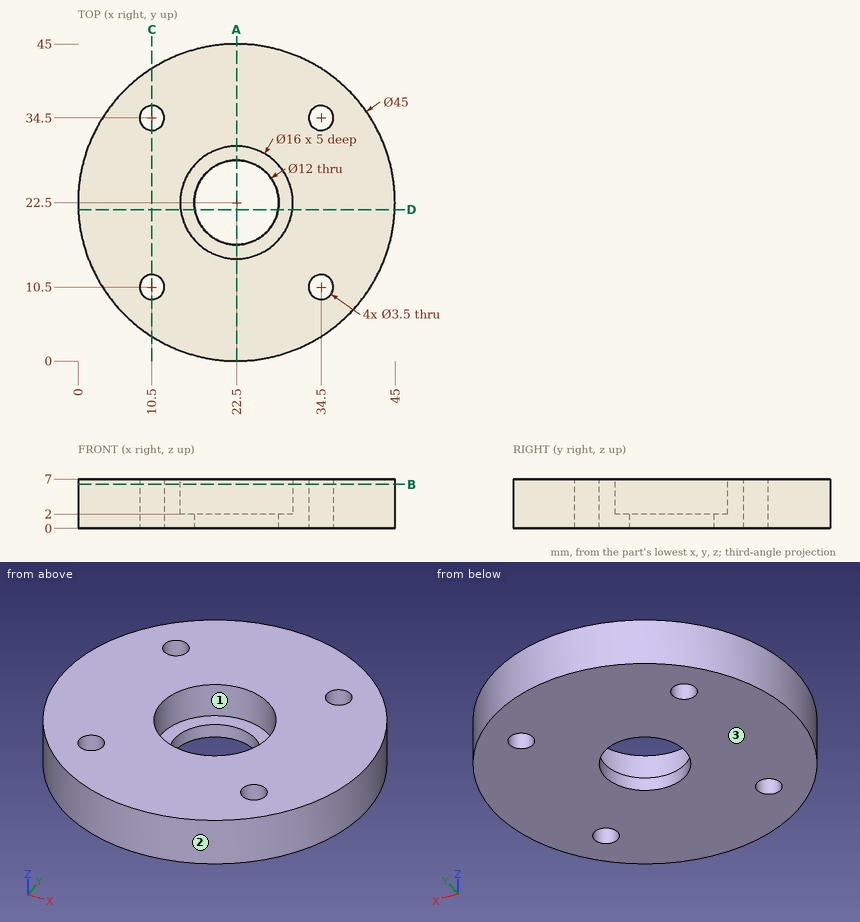
Print and shaded views of the part. All mm, measured from the part's lowest x, y and z. Coordinates: 2 decimals unless noted, no trailing zeros. Loops run counter-clockwise (first coordinate to the right, second up) from the corner with the lowest first, then second, coordinate; pieces in that order, holes last. Notation, with made-up numbers: (78.25, -9.75) - (131.25, -9.75) arc R25 cw to (131.25, 24.25) - close; hole circle Ø3 at (-37, 9). An arc over 180 degrees is marked (long way). Write item = value, one per line. Start each with the question number.
Item 1: Wall check: probe 1 along Y at (x, z) = (10.5, 2.25); probe 2 along Y at (x, z) = (9.5, 2.75); probe 3 along X at (y, z) = (33, 5). Give the ranges that are in metal, low to high. Write a range as [from, to].
Item 2: Saw through at C-C, the plane x = 10.5. List the corners of the cut face in (y, z).
Item 3: Saw through at A-A, the plane x = 22.5. List the corners of the cut face in (y, z), then the cut area to 3 significant figures.
Item 4: Saw through at D-D, the plane y = 21.5. List the corners of the cut face in (x, z), then the cut area to 3 significant figures.
Item 5: Saw through at B-B, the plane z = 6.25. List the corners of the cut face in (x, y), then the cut area to 3 significant figures.
Item 6: Pull direction X, two halves, no side cores. Call the marked faces 1, 2 and 3: +X half, -X half, draft (parallel to the pull), parting line (faces both ways), or undercut.
Item 7: Drop flat-ended pins along their axis: pin 1 Ø2 at (x, y) = (34.5, 34.5) entering from -Z; pin 2 Ø4 at (x, z) = (16, 6) entering from -Y; pin 3 Ø2 at (y, z) = (35, 2) entering from +X. Give the stop position or say it passes through.
Answers:
q1.probe_1 = [3.47, 8.75], [12.25, 32.75], [36.25, 41.53]
q1.probe_2 = [4.14, 9.06], [11.94, 33.06], [35.94, 40.86]
q1.probe_3 = [2.6, 9.6], [11.4, 33.6], [35.4, 42.4]
q2.outline = (3.47, 0) - (8.75, 0) - (8.75, 7) - (3.47, 7) - close; (12.25, 0) - (32.75, 0) - (32.75, 7) - (12.25, 7) - close; (36.25, 0) - (41.53, 0) - (41.53, 7) - (36.25, 7) - close
q3.outline = (0, 0) - (16.5, 0) - (16.5, 2) - (14.5, 2) - (14.5, 7) - (0, 7) - close; (28.5, 0) - (45, 0) - (45, 7) - (30.5, 7) - (30.5, 2) - (28.5, 2) - close
q3.area = 211 mm2
q4.outline = (0.02, 0) - (16.58, 0) - (16.58, 2) - (14.56, 2) - (14.56, 7) - (0.02, 7) - close; (28.42, 0) - (44.98, 0) - (44.98, 7) - (30.44, 7) - (30.44, 2) - (28.42, 2) - close
q4.area = 212 mm2
q5.outline = circle Ø45 at (22.5, 22.5); hole circle Ø3.5 at (10.5, 10.5); hole circle Ø3.5 at (10.5, 34.5); hole circle Ø16 at (22.5, 22.5); hole circle Ø3.5 at (34.5, 10.5); hole circle Ø3.5 at (34.5, 34.5)
q5.area = 1,350 mm2
q6.face_1 = undercut
q6.face_2 = parting line
q6.face_3 = draft
q7.pin_1 = through
q7.pin_2 = 0.45
q7.pin_3 = 41.84
